Answer from the drawing. Dimensions are ordinates in mm from the lowest x, y and z of the part. A direction names the side the tool comes from. Coordinates: 2 decimals unless noted, no trailing zeros. Order: outer loops, then holes, each group sorted by start corner. A loop starts at its lowest first (then second) coordinate and runs counter-clockwise, first axis right, second up. Notation, with made-up numbers: (-25, -26.75) - (-1, -26.75) arc R24 ccw to (-1, -12.75) - close; hole circle Ø9 at (-23, 13). An arc over 180 degrees is marked (long way). Answer as a JSON object with one key per item and string values. Group by question number.
1) Each of these flat-tipped pins is pushed along its axis until it touches: P1, Ø1.5, axis at y = 13, z = 11.5, coming from the +X side; P2, Ø2.5, axis at x = 2, y = 2, coming from the +Z side; P3, Ø1.8, axis at x = 36, y = 36, coming from the +Z side; P4, Ø2, axis at y = 15, z = 16.5, coming from the -X side. Where does it stop, or does it pass through?
2) Section D-D (x = 19) is taken. Give the vertices of the cut face in (y, z).
3) Section C-C (z = 2) is taken. Count the separate pieces of the cut face and the enclosed holes in it, plus the area to 3 significant figures.
4) Section A-A (x = 33) is taken. Give the vertices of the cut face in (y, z), plus the area to 3 significant figures.
5) Find the intervals of material crossed by line 1 along Y through (x, z) = (33, 2.65); line 2 along X through (y, z) = (36, 1.8), in increasing order.
6) A tool of negligible diameter and unlimited length cuts with its end or side. For the marked faces 1 and 2, from which of +Z, -Z, +X, -X, +Y, -Y can it reach the whole face along a straight path? Write none if from no direction.
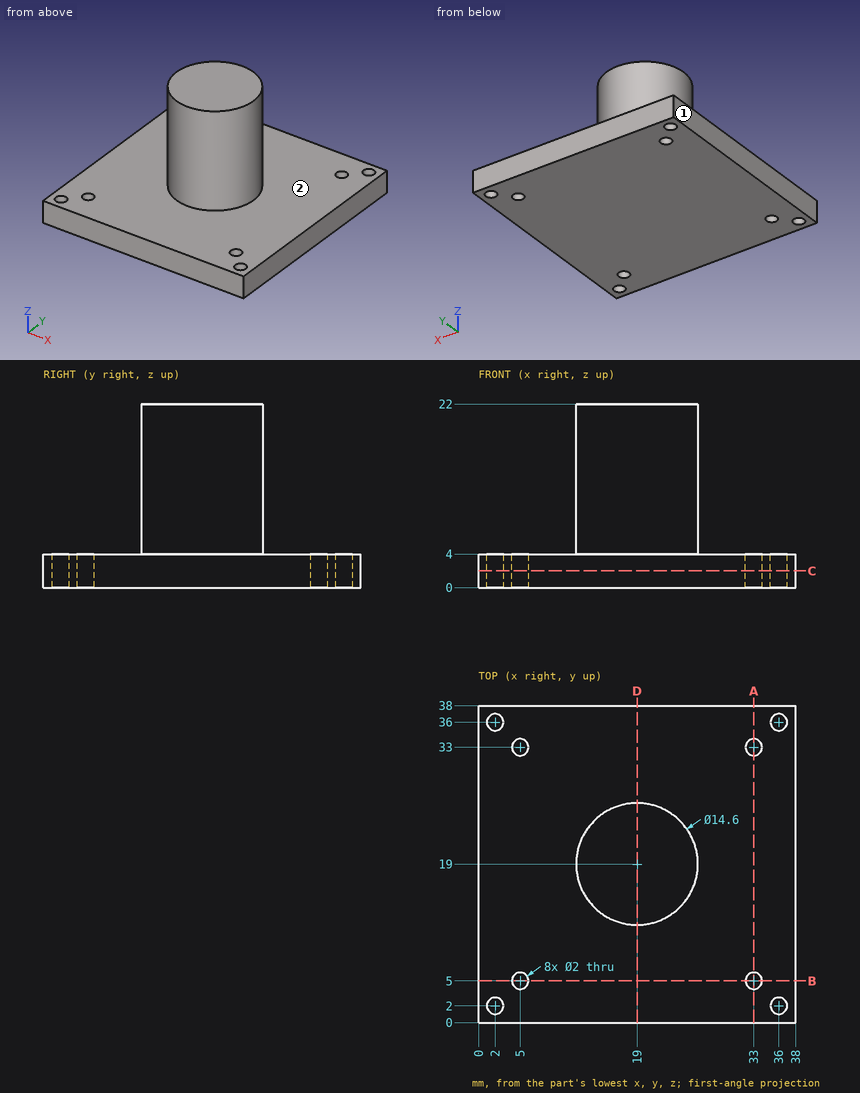
Report:
{
 "1": {"P1": "stops at x = 24.07", "P2": "stops at z = 4", "P3": "passes through", "P4": "stops at x = 12.34"},
 "2": {"outline": "(0, 0) - (38, 0) - (38, 4) - (26.3, 4) - (26.3, 22) - (11.7, 22) - (11.7, 4) - (0, 4) - close"},
 "3": {"separate pieces": "1", "enclosed holes": "8", "area": "1,420 mm²"},
 "4": {"outline": "(0, 0) - (4, 0) - (4, 4) - (0, 4) - close; (6, 0) - (32, 0) - (32, 4) - (6, 4) - close; (34, 0) - (38, 0) - (38, 4) - (34, 4) - close", "area": "136 mm²"},
 "5": {"line 1": "y = 0 to 4, 6 to 32, 34 to 38", "line 2": "x = 0 to 1, 3 to 35, 37 to 38"},
 "6": {"face 1": "+Z, -Z, -X, +Y, -Y", "face 2": "+Z"}
}
